from build123d import *

# Parameters (mm, degrees)
CUT_EXTRUDE2_DEPTH      = 63.261545114
CUT_EXTRUDE2_DEPTH_BACK = 63.261545114
SKETCH5_R               = 5
CUT_EXTRUDE3_DEPTH      = 63.060454569
CUT_EXTRUDE3_DEPTH_BACK = 63.060454569
SKETCH6_R               = 5


with BuildPart() as part:
    # Sketch2 → Revolve1 (revolve)
    with BuildSketch(Plane.XY, mode=Mode.PRIVATE) as revolve1_sk:
        Polygon((22, -42), (32.5, 0), (26.315341562, 0), (18.815341562, -30), (11.25, -30), (11.25, -42), align=None)
    revolve(revolve1_sk.sketch.rotate(Axis((0, 41.438546828, 0), (0, -1, 0)), 90), axis=Axis((0, 41.438546828, 0), (0, -1, 0)))

    # Sketch5 → Cut-Extrude2 (cut, two sides: drawn at the far end of the back side and taken through both)
    with BuildSketch(Plane.XY.offset(-CUT_EXTRUDE2_DEPTH_BACK)):
        Circle(SKETCH5_R)
    extrude(amount=CUT_EXTRUDE2_DEPTH + CUT_EXTRUDE2_DEPTH_BACK, mode=Mode.SUBTRACT)

    # Sketch6 → Cut-Extrude3 (cut, two sides: drawn at the far end of the back side and taken through both)
    with BuildSketch(Plane(origin=(0, 0, 0), x_dir=(0, 0, -1), z_dir=(1, 0, 0)).offset(-CUT_EXTRUDE3_DEPTH_BACK)):
        Circle(SKETCH6_R)
    extrude(amount=CUT_EXTRUDE3_DEPTH + CUT_EXTRUDE3_DEPTH_BACK, mode=Mode.SUBTRACT)


solid = part.part
Build history of the part. All positions in model axes, mm. Round coordinates to 2 decimals unless told otherwise and drop trailing zeros. Write each loop counter-clockwise with the first axis right and the second up, starting at its lowest first coordinate (ties: lowest second). Pieces come first, ordered by that corner, then holes. Notation, with made-up numbers: M 23,53.5 L 28,53.5 A3 ccw 28,57.5 Z; hole C -14.75,-18.5 d4. An arc over 180 degrees is marked long. Answer as a JSON object with one key per item and string values. Group by question number.
(1) Cut at B-B (x = 0). Give the cut face in (y, z), and give its area (3 significant figures).
(2) Cut at C-C (y = -4). Give the cut face in (x, z).
(3) Mould opens along Z. For faces 1 (the flat face through (9, -42, -9)), 2 (the conical face through (23.206, -25.373, 12.07)), 3 (the flat face through (8.1, -30, 8.1)), 4 (the cylindrical face through (29, -5, 0)) say: pulls with the +Z half, pulls with the -Z half, needs draft (parallel to the pull), parting line crosses it, or undercut.
(4) Drill centre lines: L1, parallel to X at y = -36.5, z = 0 (3 decimals); L2, parallel to X at y = -37.75, z = 0; L3, parallel to Y at x = 9, z = -8.5. Where is each one in solid material? Low to high.
(5) Cut at D-D (y = -23). Give the cut face in (x, z), and give its area (3 significant figures).
(6) Cut at A-A (z = 0). Give the cut face in (x, y), and give its area (3 significant figures).
(7) Flat gauge pins, fed straight in: pin 1 (5 mm diameter, centred on x = 18.5, y = -15.5, fed in from -Z); pin 2 (4 mm diameter, centred on x = -16, y = -6.5, fed in from +Z); pin 3 (2 mm diameter, centred on y = -19.5, z = 17, fed in from -X); pin 4 (13.5 mm diameter, centred on x = 0, z = 0, fed in from -Y). Where does each tip first touch, or does it go through?
Responses:
{
 "1": {"outline": "M -42,-22 L -5,-31.25 L -5,-25.07 L -30,-18.82 L -30,-11.25 L -42,-11.25 Z; M -42,11.25 L -30,11.25 L -30,18.82 L -5,25.07 L -5,31.25 L -42,22 Z", "area": "603 mm2"},
 "2": {"outline": "M -31.36,-3 A31.5 ccw -3,-31.36 L -3,-25.14 A25.32 cw -25.14,-3 Z; M -31.36,3 L -25.14,3 A25.32 cw -3,25.14 L -3,31.36 A31.5 ccw Z; M 3,-31.36 A31.5 ccw 31.36,-3 L 25.14,-3 A25.32 cw 3,-25.14 Z; M 3,25.14 A25.32 cw 25.14,3 L 31.36,3 A31.5 ccw 3,31.36 Z"},
 "3": {"face 1": "needs draft", "face 2": "parting line crosses it", "face 3": "undercut", "face 4": "undercut"},
 "4": {"L1": "x = -23.375 to -11.25, 11.25 to 23.375", "L2": "x = -23.06 to -11.25, 11.25 to 23.06", "L3": "y = -42 to -30"},
 "5": {"outline": "C 0,0 d53.5; hole C 0,0 d41.13", "area": "919 mm2"},
 "6": {"outline": "M -31.25,-5 L -22,-42 L -11.25,-42 L -11.25,-30 L -18.82,-30 L -25.07,-5 Z; M 11.25,-42 L 22,-42 L 31.25,-5 L 25.07,-5 L 18.82,-30 L 11.25,-30 Z", "area": "603 mm2"},
 "7": {"pin 1": "stops at z = -23.9", "pin 2": "stops at z = 27.66", "pin 3": "stops at x = -22.58", "pin 4": "passes through"}
}
